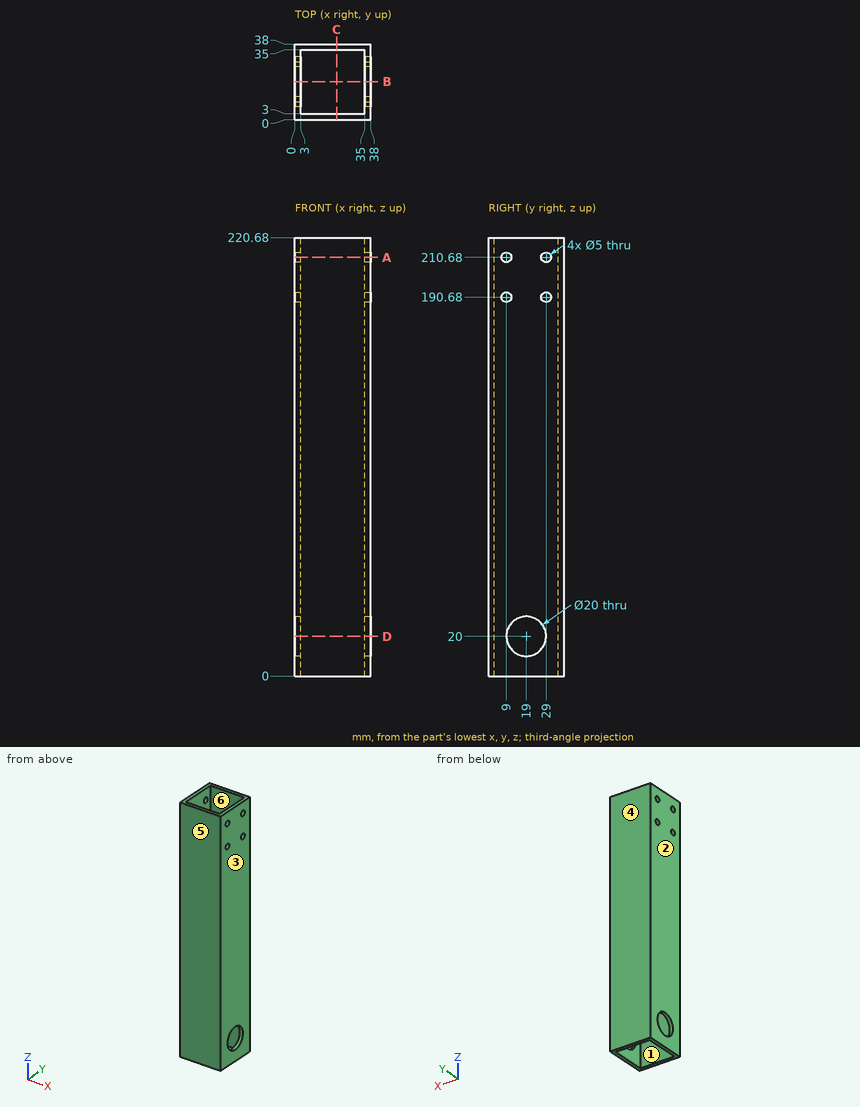
Part print with two shaded views. Sizes in mm from the minimum x, y, z corner. A direction names the side the tool comes from. Round coordinates to 2 decimals unless told otherwise and drop trailing zeros. Order: outer loops, then holes, each group sorted by start corner. A loop starts at its lowest first (then second) coordinate and runs counter-clockwise, first axis right, second up. Notation, with made-up numbers: (2.5, 39.5) -> (15.5, 39.5) arc R23 ccw to (15.5, 72.5) -> close; hole circle Ø7 at (-30, 24.5). An arc over 180 degrees is marked (long way). Use one line per item in the form item = value.
Item 1: Cut at D-D, the plane z = 20. Write the cut outline in (x, y).
Returned:
outline = (0, 0) -> (38, 0) -> (38, 9) -> (35, 9) -> (35, 3) -> (3, 3) -> (3, 9) -> (0, 9) -> close; (0, 29) -> (3, 29) -> (3, 35) -> (35, 35) -> (35, 29) -> (38, 29) -> (38, 38) -> (0, 38) -> close
Item 2: Flat gauge pin, fed straight in: pin 1 Ø12 at (y, z) = (19, 20) entering from -X. Where does the tip first touch, or does it go through?
Returned:
pin_1 = through
Item 3: Cut at C-C, the plane x = 21. Write the cut outline in (y, z), and give its area (3 significant figures).
Returned:
outline = (0, 0) -> (3, 0) -> (3, 220.68) -> (0, 220.68) -> close; (35, 0) -> (38, 0) -> (38, 220.68) -> (35, 220.68) -> close
area = 1,320 mm^2
Item 4: Cut at A-A, the plane z = 210.68. Write the cut outline in (x, y), and give its area (3 significant figures).
Returned:
outline = (0, 0) -> (38, 0) -> (38, 6.5) -> (35, 6.5) -> (35, 3) -> (3, 3) -> (3, 6.5) -> (0, 6.5) -> close; (0, 11.5) -> (3, 11.5) -> (3, 26.5) -> (0, 26.5) -> close; (0, 31.5) -> (3, 31.5) -> (3, 35) -> (35, 35) -> (35, 31.5) -> (38, 31.5) -> (38, 38) -> (0, 38) -> close; (35, 11.5) -> (38, 11.5) -> (38, 26.5) -> (35, 26.5) -> close
area = 360 mm^2
Item 5: Cut at B-B, the plane y = 19. Write the cut outline in (x, z).
Returned:
outline = (0, 0) -> (3, 0) -> (3, 10) -> (0, 10) -> close; (0, 30) -> (3, 30) -> (3, 220.68) -> (0, 220.68) -> close; (35, 0) -> (38, 0) -> (38, 10) -> (35, 10) -> close; (35, 30) -> (38, 30) -> (38, 220.68) -> (35, 220.68) -> close
Item 6: Pull direction X, two halves, no side cores. Call the marked faces 1, 2, 3 and 4: released by +X, released by -X, zero draft, split by the parting line, or undercut.
Returned:
face_1 = undercut
face_2 = released by -X
face_3 = released by +X
face_4 = zero draft
Item 7: Tool access for the marked faces 5 and 6: list every direction of +Z, -Z, +X, -X, +Y, -Y with a clear straight run to the whole face (end or side of a thin tool).
Returned:
face_5 = +Z, -Z, +X, -X, -Y
face_6 = +Z, -Z
Item 8: Drill centre lines: line 1 (Y direction, x = 36.2, z = 190.68); line 2 (Y direction, x = 29.5, z = 31). Where is each one in solid material? Low to high.
Returned:
line_1 = 0 to 6.5, 11.5 to 26.5, 31.5 to 38
line_2 = 0 to 3, 35 to 38
